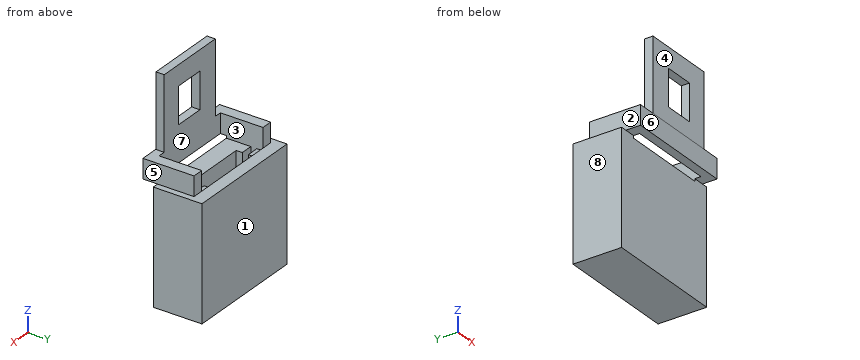
```python
from build123d import *

# Parameters (mm, degrees)
SKETCH_W        = 10
SKETCH_H        = 9.3
PAD_DEPTH       = 4
SKETCH001_W     = 9
SKETCH001_H     = 1.6
PAD001_DEPTH    = 3
SKETCH002_W     = 9
SKETCH002_H     = 1.6
PAD002_DEPTH    = 1.2
SKETCH003_W     = 7.2
SKETCH003_H     = 3.5
POCKET_DEPTH    = 1.8
POCKET001_DEPTH = 8
SKETCH005_W     = 6
SKETCH005_H     = 0.68
PAD003_DEPTH    = 6
SKETCH006_W     = 2.5
SKETCH006_H     = 3
POCKET002_DEPTH = 5


with BuildPart() as part:
    # Sketch → Pad (new body)
    with BuildSketch(Plane.XZ):
        with Locations((5, 4.65)):
            Rectangle(SKETCH_W, SKETCH_H)
    extrude(amount=PAD_DEPTH)

    # Sketch001 (on Face6 of Pad) → Pad001 (join)
    with BuildSketch(Plane.XZ.offset(4)):
        with Locations((5, 10.1)):
            Rectangle(SKETCH001_W, SKETCH001_H)
    extrude(amount=-PAD001_DEPTH)

    # Sketch002 (on Face10 of Pad001) → Pad002 (join)
    with BuildSketch(Plane.XZ.offset(4)):
        with Locations((5, 10.1)):
            Rectangle(SKETCH002_W, SKETCH002_H)
    extrude(amount=PAD002_DEPTH)

    # Sketch003 (on Face12 of Pad002) → Pocket (cut)
    with BuildSketch(Plane(origin=(0, 0, 10.9), x_dir=(-1, 0, 0), z_dir=(0, 0, 1))):
        with Locations((-5, 2.75)):
            Rectangle(SKETCH003_W, SKETCH003_H)
    extrude(amount=-POCKET_DEPTH, mode=Mode.SUBTRACT)

    # Sketch004 (on Face9 of Pocket) → Pocket001 (cut)
    with BuildSketch(Plane(origin=(0, 0, 9.1), x_dir=(-1, 0, 0), z_dir=(0, 0, 1))):
        Polygon((-8.6, 1.5), (-7.6, 1.5), (-7.6, 1), (-2.4, 1), (-2.4, 1.5), (-1.4, 1.5), (-1.4, 2), (-2.4, 2), (-2.4, 2.5), (-7.85, 2.5), (-7.85, 2), (-8.6, 2), align=None)
    extrude(amount=-POCKET001_DEPTH, mode=Mode.SUBTRACT)

    # Sketch005 (on Face21 of Pocket001) → Pad003 (join)
    with BuildSketch(Plane(origin=(0, 0, 10.9), x_dir=(-1, 0, 0), z_dir=(0, 0, 1))):
        with Locations((-5, 4.84)):
            Rectangle(SKETCH005_W, SKETCH005_H)
    extrude(amount=PAD003_DEPTH)

    # Sketch006 (on Face30 of Pad003) → Pocket002 (cut)
    with BuildSketch(Plane.XZ.offset(5.18)):
        with Locations((5.05, 13.75)):
            Rectangle(SKETCH006_W, SKETCH006_H)
    extrude(amount=-POCKET002_DEPTH, mode=Mode.SUBTRACT)


solid = part.part
```
For this review, take the finished solid that the model builds, in its own axes (mm). Face numbers are marked on the shaded views. A direction names the side the tool comes from. Round coordinates to 2 decimals unless told otherwise and drop trailing zeros. Write each loop counter-clockwise with the first axis right and the second up, starting at its lowest first coordinate (ties: lowest second). Pieces come first, ordered by that corner, then holes.
1) Machinability: for the marked faces 1, 2, 3, 4 and 5, which of the approach directions +Z, -Z, +X, -X, +Y, -Y give a long, thin tool a straight path to every point of the face, cutting with its end or side? Answer none if there is none.
Answer below:
face 1: +Z, -Z, +X, -X, +Y
face 2: +Z, -X, +Y, -Y
face 3: +Z
face 4: +Z, +X, -X, -Y
face 5: +Z, +X, +Y, -Y
2) Take a section at C-C on y = -3.1. Give the boundary of the cut face in (x, z).
Answer below:
outline: (0, 0) - (10, 0) - (10, 9.3) - (9.5, 9.3) - (9.5, 10.9) - (8.6, 10.9) - (8.6, 9.1) - (1.4, 9.1) - (1.4, 10.9) - (0.5, 10.9) - (0.5, 9.3) - (0, 9.3) - close
3) For line 1 along Y through (x, z) = (6.5, 4.5); line 2 along X through (y, z) = (-1.05, 10.5); line 3 along X through (y, z) = (-2.15, 5.5), list the stretches that pass through material, from the lowest coordinate up.
Answer below:
line 1: y = -4 to -2.5, -1 to 0
line 2: x = 0.5 to 1.4, 8.6 to 9.5
line 3: x = 0 to 2.4, 7.85 to 10
4) Mouldability with a two-part tool opening along X and no side actions: class the marked faces 6, 7 and 8 as +X half, -X half, draft (parallel to the pull), parting line (faces both ways), or undercut.
Answer below:
face 6: draft
face 7: undercut
face 8: -X half
5) Insertion check: pin 1 Ø1.6 at (x, y) = (4.5, -1.5) entering from +Z; pin 2 Ø3 at (x, z) = (2.5, 4) entering from -Y; pin 3 Ø1.3 at (y, z) = (-3.5, 10) entering from -X. Each pin has a flat end and moves straight along its axis. Give the tip position at first contact, or say it passes through.
Answer below:
pin 1: stops at z = 9.3
pin 2: stops at y = -4
pin 3: stops at x = 0.5
6) Take a section at B-B on z = 12.5. Give the boundary of the cut face in (x, y).
Answer below:
outline: (2, -5.18) - (3.8, -5.18) - (3.8, -4.5) - (2, -4.5) - close; (6.3, -5.18) - (8, -5.18) - (8, -4.5) - (6.3, -4.5) - close
7) Take a section at D-D on z = 8.75. Give the boundary of the cut face in (x, y), then the cut area to 3 significant figures.
Answer below:
outline: (0, -4) - (10, -4) - (10, 0) - (0, 0) - close; hole (1.4, -2) - (2.4, -2) - (2.4, -2.5) - (7.85, -2.5) - (7.85, -2) - (8.6, -2) - (8.6, -1.5) - (7.6, -1.5) - (7.6, -1) - (2.4, -1) - (2.4, -1.5) - (1.4, -1.5) - close
area: 31.1 mm2
